Verification items for the finished model (mm, model axes). Face numbers are marked on the shaded views. A direction names the side the tool comes from. Round coordinates to 2 decimals unless told otherwise and drop trailing zeros. Order: outer loops, then holes, each group sorted by start corner. A loop starts at its lowest first (then second) coordinate and runs counter-clockwise, first axis right, second up. Notation, with made-up numbers: (83.25, 71.5) -> (118.25, 71.5) arc R9 cw to (118.25, 85.5) -> close; hole circle Ø10 at (44.25, 17). An arc over 180 degrees is marked (long way). Put each result on its own line as item: value.
```python
from build123d import *

# Parameters (mm, degrees)
SKETCH1_W                   = 20
SKETCH1_H                   = 540
BOSS_EXTRUDE1_DEPTH         = 150
SKETCH2_W                   = 540
SKETCH2_H                   = 20
BOSS_EXTRUDE2_DEPTH         = 36
M10_TAPPED_HOLE1_AT_2_COUNT = 2
M10_TAPPED_HOLE1_AT_2_PITCH = 80
M10_TAPPED_HOLE1_AT_3_COUNT = 2
M10_TAPPED_HOLE1_AT_3_PITCH = 160


with BuildPart() as part:
    # Sketch1 → Boss-Extrude1 (new body)
    with BuildSketch(Plane(origin=(0, 0, 0), x_dir=(1, 0, 0), z_dir=(0, 1, 0))):
        with Locations((10, 0)):
            Rectangle(SKETCH1_W, SKETCH1_H)
    extrude(amount=BOSS_EXTRUDE1_DEPTH)

    # Sketch2 → Boss-Extrude2 (add)
    with BuildSketch(Plane(origin=(0, 0, 0), x_dir=(0, 0, -1), z_dir=(1, 0, 0))):
        with Locations((0, 10)):
            Rectangle(SKETCH2_W, SKETCH2_H)
    extrude(amount=-BOSS_EXTRUDE2_DEPTH)

    # Sketch6 → M10 Tapped Hole1 (revolve, cut)
    with BuildSketch(Plane(origin=(-16, 20, -80), x_dir=(0, 0, 1), z_dir=(1, 0, 0))):
        Polygon((0, 0), (0, 27.5), (4.25, 24.946342369), (4.25, 0.775), (5.025, 0), align=None)
    m10_tapped_hole1 = revolve(axis=Axis((-16, 26.35, -80), (0, -1, 0)), mode=Mode.SUBTRACT)

    # M10 Tapped Hole1 at 2: M10 Tapped Hole1 ×2
    with Locations(*[(0, 0, -i * M10_TAPPED_HOLE1_AT_2_PITCH) for i in range(1, M10_TAPPED_HOLE1_AT_2_COUNT)]):
        add(m10_tapped_hole1, mode=Mode.SUBTRACT)

    # M10 Tapped Hole1 at 3: M10 Tapped Hole1 ×2
    with Locations(*[(0, 0, -i * M10_TAPPED_HOLE1_AT_3_PITCH) for i in range(1, M10_TAPPED_HOLE1_AT_3_COUNT)]):
        add(m10_tapped_hole1, mode=Mode.SUBTRACT)

    # Mirror1: M10 Tapped Hole1 across plane
    add(m10_tapped_hole1.mirror(Plane.XY), mode=Mode.SUBTRACT)

    # Mirror1 copy 1 sketch → Mirror1 copy 1 (revolve, cut)
    with BuildSketch(Plane(origin=(-16, 20, 160), x_dir=(0, 0, -1), z_dir=(1, 0, 0))):
        Polygon((0, 0), (0, -27.5), (4.25, -24.946342369), (4.25, -0.775), (5.025, 0), align=None)
    revolve(axis=Axis((-16, 26.35, 160), (0, 1, 0)), mode=Mode.SUBTRACT)

    # Mirror1 copy 2 sketch → Mirror1 copy 2 (revolve, cut)
    with BuildSketch(Plane(origin=(-16, 20, 240), x_dir=(0, 0, -1), z_dir=(1, 0, 0))):
        Polygon((0, 0), (0, -27.5), (4.25, -24.946342369), (4.25, -0.775), (5.025, 0), align=None)
    revolve(axis=Axis((-16, 26.35, 240), (0, 1, 0)), mode=Mode.SUBTRACT)


solid = part.part
```
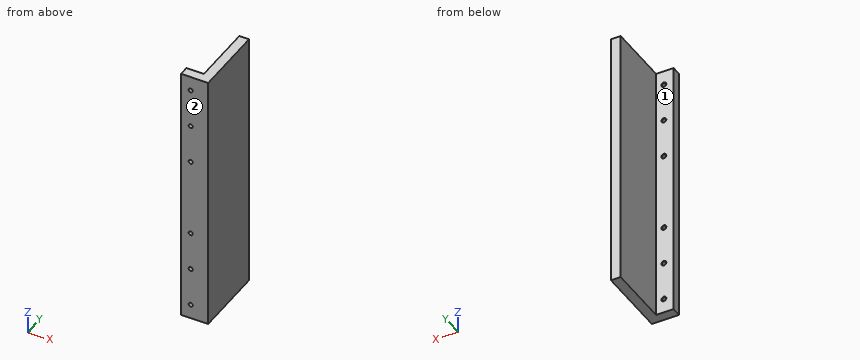
Item 1: Material ranges on line 1 along X through (y, z) = (5.25, 160); line 2 along Y through (x, z) = (-29.5, -108), recorded low to high.
Geometry check:
line 1: -36 to -20.25, -11.75 to 20
line 2: 0 to 20
Item 2: Sectioned sample at A-A, the plane x = -5.5. Record the boundary of the cut face in (y, z).
Geometry check:
outline: (0, -270) -> (20, -270) -> (20, 270) -> (0, 270) -> close
Item 3: Tool access check on the marked faces 1 and 2. Record the directions out of +Z, -Z, +X, -X, +Y, -Y that give a thin tool (end or side, any length) a straight path to the whole face; none if there is none.
Geometry check:
face 1: +Z, -Z, -X, +Y
face 2: +Z, -Z, +X, -X, -Y
Item 4: Depth check by flat-ended pin: pin 1 Ø6 at (y, z) = (89.5, -177.5) entering from -X; pin 2 Ø10 at (x, z) = (-16, 240) entering from +Y (3 decimals). Enter the tip coordinate at first touch or a pass-through.
Geometry check:
pin 1: x = 0
pin 2: y = 19.975
